Input: part model. Units: mm. Frame: model coordinates. A direction names the side the tool comes from. Coordinates: 2 decimals unless noted, no trailing zeros. Order: outer loops, then holes, each group sorted by start corner. A loop starts at its lowest first (then second) coordinate and runs counter-clockwise, first axis right, second up. Notation, with made-up numbers: (-40, -36.5) - (5, -36.5) arc R21 ccw to (5, -10.5) - close; hole circle Ø7 at (1.25, 85). An arc over 180 degrees is marked (long way). Answer as CSV lines item,"result". Start each with the question number.
Item 1: Section B-B (y = -66.5). State how many separate pieces and enclosed holes the cut face has, and give its area (3 significant figures).
Item 2: Section A-A (x = 2). Output: boundary loops of the cut face in (y, z), and give its area (3 significant figures).
Item 3: Material intervals for line 1 along Z through (x, y) = (-16, -205); line 2 along Z through (x, y) = (-7.5, -65.5); line 3 along X through (y, z) = (-230.5, -15.5), sorted ascending.
Item 4: Access query for faces 1 (the flat face through (19, -123, 3.902)), 2 (the flat face through (21.97, -123, -15)), 3 (the flat face through (-5.53, -123, 19)), 4 (the flat face through (11.97, -123, -1)), 5 (the flat face through (-23.03, -123, -14)). Directions: +Z, -Z, +X, -X, +Y, -Y. A direction counts if a zero-diameter tool reaches every point of the face in a straight line with its end or side. Return the directions, or none.
Item 5: First-contact query: pin 1 (11 mm diameter, centred on x = -0.53, z = -1.1, fed in from -Y); pin 2 (4.5 mm diameter, centred on x = -1, y = -185.5, fed in from +Z). Flat tips, straight axial feed; report the tip coordinate or a pass-through.
from build123d import *

# Parameters (mm, degrees)
F0_R     = 4.5
F0_R_2   = 6
F1_DEPTH = 250
F2_R     = 1
F3_R     = 0.5
F4_SIZE  = 0.5


with BuildPart() as f1:
    # F0 (on Front) → F1 (new body)
    with BuildSketch(Plane.XZ):
        Polygon((4.469697, -23.598485), (21.969697, -23.598485), (21.969697, -6.098485), (16.969697, -6.098485), (16.969697, -8.598485), (11.969697, -8.598485), (11.969697, 6.401515), (16.969697, 6.401515), (16.969697, 3.901515), (21.969697, 3.901515), (21.969697, 21.401515), (4.469697, 21.401515), (4.469697, 16.401515), (6.969697, 16.401515), (6.969697, 11.401515), (-8.030303, 11.401515), (-8.030303, 16.401515), (-5.530303, 16.401515), (-5.530303, 21.401515), (-23.030303, 21.401515), (-23.030303, 3.901515), (-18.030303, 3.901515), (-18.030303, 6.401515), (-13.030303, 6.401515), (-13.030303, -8.598485), (-18.030303, -8.598485), (-18.030303, -6.098485), (-23.030303, -6.098485), (-23.030303, -23.598485), (-5.530303, -23.598485), (-5.530303, -18.598485), (-8.030303, -18.598485), (-8.030303, -13.598485), (6.969697, -13.598485), (6.969697, -18.598485), (4.469697, -18.598485), align=None)
        with Locations((-15.530303, -16.098485)):
            Circle(F0_R, mode=Mode.SUBTRACT)
        with Locations((14.469697, -16.098485)):
            Circle(F0_R, mode=Mode.SUBTRACT)
        with Locations((-0.530303, -1.098485)):
            Circle(F0_R_2, mode=Mode.SUBTRACT)
        with Locations((-15.530303, 13.901515)):
            Circle(F0_R, mode=Mode.SUBTRACT)
        with Locations((14.469697, 13.901515)):
            Circle(F0_R, mode=Mode.SUBTRACT)
    extrude(amount=F1_DEPTH)

    # F2
    f2_edges = [f1.edges().sort_by_distance(p)[0] for p in [
        (21.969697, -125, 21.401515),
        (21.969697, -125, -23.598485),
        (-23.030303, -125, -23.598485),
        (-23.030303, -125, 21.401515),
    ]]
    fillet(f2_edges, radius=F2_R)

    # F3
    f3_edges = [f1.edges().sort_by_distance(p)[0] for p in [
        (-18.030303, -125, -6.098485),
        (-18.030303, -125, 3.901515),
        (-5.530303, -125, -18.598485),
        (4.469697, -125, -18.598485),
        (16.969697, -125, -6.098485),
        (-5.530303, -125, 16.401515),
        (4.469697, -125, 16.401515),
        (16.969697, -125, 3.901515),
    ]]
    fillet(f3_edges, radius=F3_R)

    # F4
    f4_edges = [f1.edges().sort_by_distance(p)[0] for p in [
        (21.969697, -125, -6.098485),
        (21.969697, -125, 3.901515),
        (4.469697, -125, 21.401515),
        (-5.530303, -125, 21.401515),
        (-23.030303, -125, 3.901515),
        (-23.030303, -125, -6.098485),
        (4.469697, -125, -23.598485),
        (-5.530303, -125, -23.598485),
    ]]
    chamfer(f4_edges, length=F4_SIZE)


solid = f1.part
Determined:
1,separate pieces,"1"
1,enclosed holes,"5"
1,area,"1,160 mm^2"
2,outline,"(-250, -13.6) - (0, -13.6) - (0, -6.54) - (-250, -6.54) - close; (-250, 4.34) - (0, 4.34) - (0, 11.4) - (-250, 11.4) - close"
2,area,"3,530 mm^2"
3,line 1,"z = -23.6 to -20.57, -11.62 to -8.6, 6.4 to 9.43, 18.38 to 21.4"
3,line 2,"z = -23.6 to -18.6, -13.6 to 11.4, 16.4 to 21.4"
3,line 3,"x = -23.03 to -19.99, -11.07 to -8.03, 6.97 to 10.01, 18.93 to 21.97"
4,face 1,"+X, +Y, -Y"
4,face 2,"+Z, -Z, +X, +Y, -Y"
4,face 3,"+Z, +Y, -Y"
4,face 4,"+Y, -Y"
4,face 5,"+Z, -Z, -X, +Y, -Y"
5,pin 1,"passes through"
5,pin 2,"stops at z = 11.4"
